from build123d import *

# Parameters (mm, degrees)
SKETCH_W      = 60
SKETCH_H      = 3
PAD_DEPTH     = 35
SKETCH001_R   = 1.5
SKETCH001_R_2 = 2
SKETCH001_R_3 = 2.25
SKETCH001_R_4 = 1
SKETCH001_W   = 4
SKETCH001_H   = 7
POCKET_DEPTH  = 3


with BuildPart() as part:
    # Sketch → Pad (new body)
    with BuildSketch(Plane.XY):
        with Locations((30, 1.5)):
            Rectangle(SKETCH_W, SKETCH_H)
    extrude(amount=PAD_DEPTH)

    # Sketch001 → Pocket (cut)
    with BuildSketch(Plane.XZ):
        with Locations((22, 10)):
            Circle(SKETCH001_R)
        with Locations((28, 10)):
            Circle(SKETCH001_R_2)
        with Locations((22, 16)):
            Circle(SKETCH001_R_2)
        with Locations((16, 10)):
            Circle(SKETCH001_R_2)
        with Locations((22, 4)):
            Circle(SKETCH001_R_2)
        with Locations((5, 30)):
            Circle(SKETCH001_R_3)
        with Locations((55, 30)):
            Circle(SKETCH001_R_3)
        with Locations((14, 30)):
            Circle(SKETCH001_R_4)
        with Locations((18, 30)):
            Circle(SKETCH001_R_4)
        with Locations((26, 30)):
            Circle(SKETCH001_R_4)
        with Locations((30, 30)):
            Circle(SKETCH001_R_4)
        with Locations((34, 30)):
            Circle(SKETCH001_R_4)
        with Locations((42, 30)):
            Circle(SKETCH001_R_4)
        with Locations((46, 30)):
            Circle(SKETCH001_R_4)
        with Locations((22, 30)):
            Rectangle(SKETCH001_W, SKETCH001_H)
        with Locations((38, 30)):
            Rectangle(SKETCH001_W, SKETCH001_H)
    extrude(amount=-POCKET_DEPTH, mode=Mode.SUBTRACT)


solid = part.part
Geometry check sheet. Reference: the model listing, model coordinates, mm. A direction names the side the tool comes from. Coordinates: 2 decimals unless noted, no trailing zeros. Write each loop counter-clockwise with the first axis right and the second up, starting at its lowest first coordinate (ties: lowest second). Pieces come first, ordered by that corner, then holes. Notation, with made-up numbers: (52, 43.5) -> (96, 43.5) arc R13 ccw to (96, 53.5) -> close; hole circle Ø3 at (-30.5, 43.5). An arc over 180 degrees is marked (long way). One line per question, with ' | ' between items.
1. Cross-section at A-A on x = 28. Record the cut outline in (y, z), and give its area (3 significant figures).
Answers:
outline: (0, 0) -> (3, 0) -> (3, 8) -> (0, 8) -> close; (0, 12) -> (3, 12) -> (3, 35) -> (0, 35) -> close | area: 93.0 mm²
2. Thickness scan on probe 1 along Z at (x, y) = (22, 1.75); probe 2 along Z at (x, y) = (28, 0.95); probe 3 along Z at (x, y) = (39.5, 1.45). Record the ranges inside material, lowest first. Write a range as from..to.
Answers:
probe 1: z = 0..2, 6..8.5, 11.5..14, 18..26.5, 33.5..35 | probe 2: z = 0..8, 12..35 | probe 3: z = 0..26.5, 33.5..35
3. Draft check along Z on faces 3 (the cylindrical face through (20.4, 1.5, 2.8)), 4 (the flat face through (30, 0, 17)). Enter one of: +Z half, -Z half, draft (parallel to the pull), parting line (faces both ways), or undercut.
Answers:
face 3: undercut | face 4: draft
4. Cross-section at C-C on y = 1.45. State how many separate pieces and enclosed holes the cut face has, and give its area (3 significant figures).
Answers:
separate pieces: 1 | enclosed holes: 16 | area: 1,930 mm²
5. Cross-section at D-D on x = 42. Record the cut outline in (y, z), and give its area (3 significant figures).
Answers:
outline: (0, 0) -> (3, 0) -> (3, 29) -> (0, 29) -> close; (0, 31) -> (3, 31) -> (3, 35) -> (0, 35) -> close | area: 99.0 mm²
6. Set-up check for faces 1 (the flat face through (0, 1, 17)), 2 (the flat face through (20, 1, 30)): record each of +Z, -Z, +X, -X, +Y, -Y from which the full face is reachable in a straight line by a thin tool's end or side.
Answers:
face 1: +Z, -Z, -X, +Y, -Y | face 2: +Y, -Y
7. Cross-section at B-B on z = 10. Record the cut outline in (x, y), and give its area (3 significant figures).
Answers:
outline: (0, 0) -> (14, 0) -> (14, 3) -> (0, 3) -> close; (18, 0) -> (20.5, 0) -> (20.5, 3) -> (18, 3) -> close; (23.5, 0) -> (26, 0) -> (26, 3) -> (23.5, 3) -> close; (30, 0) -> (60, 0) -> (60, 3) -> (30, 3) -> close | area: 147 mm²
